Geometry check sheet. Reference: the model listing, model coordinates, mm. Round coordinates to 2 decimals unless told otherwise and drop trailing zeros. Loops run counter-clockwise (first coordinate to the right, second up) from the corner with the lowest first, then second, coordinate; pieces in that order, holes last.
```python
from build123d import *

# Parameters (mm, degrees)
SKETCH1_R                                    = 10.5
SKETCH1_R_2                                  = 5
BOSS_EXTRUDE1_DEPTH                          = 3
CUT_EXTRUDE1_REACH                           = 140.687
SKETCH2_R                                    = 2
BOSS_EXTRUDE2_DEPTH                          = 3
SKETCH4_W                                    = 2
SKETCH4_H                                    = 6.5
SKETCH4_W_2                                  = 6.5
SKETCH4_H_2                                  = 2
BOSS_EXTRUDE3_DEPTH                          = 1
SKETCH5_R                                    = 2
CUT_EXTRUDE2_DEPTH                           = 10
CSK_FOR_M4_HEX_SOCKET_COUNTERSUNK_HE_2_COUNT = 2
CSK_FOR_M4_HEX_SOCKET_COUNTERSUNK_HE_2_PITCH = 16
CSK_FOR_M4_HEX_SOCKET_COUNTERSUNK_HE_3_COUNT = 2
CSK_FOR_M4_HEX_SOCKET_COUNTERSUNK_HE_3_PITCH = 16
CSK_FOR_M4_HEX_SOCKET_COUNTERSUNK_HE_4_COUNT = 2
CSK_FOR_M4_HEX_SOCKET_COUNTERSUNK_HE_4_PITCH = 22.627416998


with BuildPart() as part:
    # Sketch1 → Boss-Extrude1 (new body)
    # profile 1 of 2: a face of its own
    with BuildSketch(Plane.XY):
        with BuildLine():
            ThreePointArc((-60, 0), (-52.867640737, 28.372743309), (-33.166247904, 50))
            Line((-33.166247904, 50), (-60, 50))
            Line((-60, 50), (-60, 0))
        make_face()
    # profile 2 of 2: a face of its own
    with BuildSketch(Plane.XY):
        with BuildLine():
            ThreePointArc((0, 60), (-17.320508076, 57.445626465), (-33.166247904, 50))
            ThreePointArc((-33.166247904, 50), (-52.867640737, 28.372743309), (-60, 0))
            ThreePointArc((-60, 0), (-6.678621673, -59.627141576), (58.513200418, -13.274237334))
            Line((58.513200418, -13.274237334), (87.081101726, -13.274237334))
            Line((87.081101726, -13.274237334), (117.67766953, 17.32233047))
            ThreePointArc((117.67766953, 17.32233047), (123.096988313, 44.567085809), (100, 60))
            Line((100, 60), (0, 60))
        make_face()
        Circle(SKETCH1_R, mode=Mode.SUBTRACT)
        with Locations((100, 35)):
            Circle(SKETCH1_R_2, mode=Mode.SUBTRACT)
    extrude(amount=BOSS_EXTRUDE1_DEPTH)

    # Sketch2 → Cut-Extrude1 (cut, up to next)
    with BuildSketch(Plane.XY.offset(3), mode=Mode.PRIVATE) as cut_extrude1_sk1:
        with Locations((60, 45)):
            Circle(SKETCH2_R)
    cut_extrude1_tool1 = extrude(cut_extrude1_sk1.sketch, amount=-CUT_EXTRUDE1_REACH, mode=Mode.PRIVATE) & part.part
    # Sketch2 → Cut-Extrude1 (cut, up to next)
    with BuildSketch(Plane.XY.offset(3), mode=Mode.PRIVATE) as cut_extrude1_sk2:
        with Locations((76, 11.725762666)):
            Circle(SKETCH2_R)
    cut_extrude1_tool2 = extrude(cut_extrude1_sk2.sketch, amount=-CUT_EXTRUDE1_REACH, mode=Mode.PRIVATE) & part.part
    add(cut_extrude1_tool1.solids().sort_by_distance((60, 45, 3))[0], mode=Mode.SUBTRACT)
    add(cut_extrude1_tool2.solids().sort_by_distance((76, 11.725763, 3))[0], mode=Mode.SUBTRACT)

    # Sketch3 → Boss-Extrude2 (add)
    with BuildSketch(Plane(origin=(0, 0, 0), x_dir=(-1, 0, 0), z_dir=(0, 0, -1))):
        with BuildLine():
            Line((-30, 80), (-30, 60))
            Line((-30, 60), (0, 60))
            ThreePointArc((0, 60), (2.502176759, 59.947803225), (5, 59.791303716))
            Line((5, 59.791303716), (5, 80))
            Line((5, 80), (-30, 80))
        make_face()
    extrude(amount=-BOSS_EXTRUDE2_DEPTH)

    # Sketch4 → Boss-Extrude3 (add)
    with BuildSketch(Plane(origin=(0, 0, 0), x_dir=(-1, 0, 0), z_dir=(0, 0, -1))):
        with Locations((-12.5, 68.846087829)):
            Rectangle(SKETCH4_W, SKETCH4_H)
        with Locations((-16.75, 64.596087829)):
            Rectangle(SKETCH4_W_2, SKETCH4_H_2)
        with Locations((-12.5, 64.596087829)):
            Rectangle(SKETCH4_W, SKETCH4_H_2)
        with Locations((-8.25, 64.596087829)):
            Rectangle(SKETCH4_W_2, SKETCH4_H_2)
        with Locations((-12.5, 60.346087829)):
            Rectangle(SKETCH4_W, SKETCH4_H)
    extrude(amount=BOSS_EXTRUDE3_DEPTH)

    # Sketch5 → Cut-Extrude2 (cut)
    with BuildSketch(Plane.XY.offset(3)):
        with Locations((92, 43)):
            Circle(SKETCH5_R)
        with Locations((108, 43)):
            Circle(SKETCH5_R)
        with Locations((108, 27)):
            Circle(SKETCH5_R)
        with Locations((92, 27)):
            Circle(SKETCH5_R)
    extrude(amount=-CUT_EXTRUDE2_DEPTH, mode=Mode.SUBTRACT)

    # Sketch8 → CSK for M4 Hex Socket Countersunk Head Screw1 (revolve, cut)
    with BuildSketch(Plane(origin=(92, 43, 3), x_dir=(0, -1, 0), z_dir=(1, 0, 0))):
        Polygon((0, 0), (0, 4), (2.25, 4), (2.25, 2.34), (4.59, 0), align=None)
    csk_for_m4_hex_socket_countersunk_head_s = revolve(axis=Axis((92, 43, 9.35), (0, 0, -1)), mode=Mode.SUBTRACT)

    # CSK for M4 Hex Socket Countersunk He 2: CSK for M4 Hex Socket Countersunk Head Screw1 ×2
    with Locations(*[(i * CSK_FOR_M4_HEX_SOCKET_COUNTERSUNK_HE_2_PITCH, 0, 0) for i in range(1, CSK_FOR_M4_HEX_SOCKET_COUNTERSUNK_HE_2_COUNT)]):
        add(csk_for_m4_hex_socket_countersunk_head_s, mode=Mode.SUBTRACT)

    # CSK for M4 Hex Socket Countersunk He 3: CSK for M4 Hex Socket Countersunk Head Screw1 ×2
    with Locations(*[(0, -i * CSK_FOR_M4_HEX_SOCKET_COUNTERSUNK_HE_3_PITCH, 0) for i in range(1, CSK_FOR_M4_HEX_SOCKET_COUNTERSUNK_HE_3_COUNT)]):
        add(csk_for_m4_hex_socket_countersunk_head_s, mode=Mode.SUBTRACT)

    # CSK for M4 Hex Socket Countersunk He 4: CSK for M4 Hex Socket Countersunk Head Screw1 ×2
    with Locations(*[Vector(0.7071067811865472, -0.7071067811865478, 0) * (i * CSK_FOR_M4_HEX_SOCKET_COUNTERSUNK_HE_4_PITCH) for i in range(1, CSK_FOR_M4_HEX_SOCKET_COUNTERSUNK_HE_4_COUNT)]):
        add(csk_for_m4_hex_socket_countersunk_head_s, mode=Mode.SUBTRACT)


solid = part.part
```
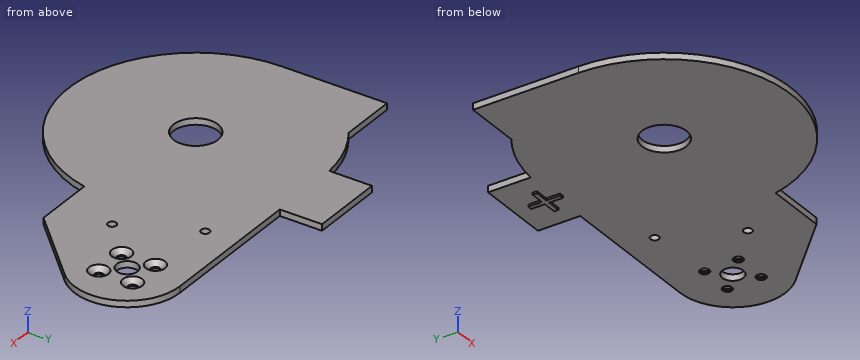
1) Sectioned sample at A-A, the plane y = 35. Record the cut outline in (x, z), then the cut area to 3 significant figures.
Report:
outline: (-60, 0) - (95, 0) - (95, 3) - (-60, 3) - close; (105, 0) - (125, 0) - (125, 3) - (105, 3) - close
area: 525 mm2
2) Sectioned sample at C-C, the plane x = 108. Record the cut outline in (y, z).
Report:
outline: (7.64, 0) - (24.75, 0) - (24.75, 0.66) - (22.41, 3) - (7.64, 3) - close; (29.25, 0) - (40.75, 0) - (40.75, 0.66) - (38.41, 3) - (31.59, 3) - (29.25, 0.66) - close; (45.25, 0) - (58.69, 0) - (58.69, 3) - (47.59, 3) - (45.25, 0.66) - close
3) Gauge pin test, flat ends, axial feed: pin 1 (1.1 mm diameter, centred on y = 70, z = -0.5, fed in from -X); pin 2 (0.5 mm diameter, centred on y = 64.5, z = -0.5, fed in from +X); pin 3 (0.8 mm diameter, centred on y = 59.5, z = -0.5, fed in from +X). Record the tip position at first contact, or that the pin passes through.
Report:
pin 1: stops at x = -5
pin 2: stops at x = 20
pin 3: stops at x = 13.5
4) Sectioned sample at B-B, the plane x = 76. Record the cut outline in (y, z), then the cut area to 3 significant figures.
Report:
outline: (-13.27, 0) - (9.73, 0) - (9.73, 3) - (-13.27, 3) - close; (13.73, 0) - (60, 0) - (60, 3) - (13.73, 3) - close
area: 208 mm2
5) Scan lines: line 1 along Y through (x, z) = (76, 1); line 2 along X through (y, z) = (27, 0.2); line 3 along Y through (x, z) = (92, 0.55). Record each from-to range of solid material in increasing order.
Report:
line 1: y = -13.27 to 9.73, 13.73 to 60
line 2: x = -60 to 89.75, 94.25 to 105.75, 110.25 to 123.69
line 3: y = -8.36 to 24.75, 29.25 to 40.75, 45.25 to 60
6) Sectioned sample at D-D, the plane y = -48. Record the cut outline in (x, z), then the cut area to 3 significant figures.
Report:
outline: (-36, 0) - (36, 0) - (36, 3) - (-36, 3) - close
area: 216 mm2
